Can you work these out from the model? Positions are in its coordinate system, mm. A direction names the side the tool comes from. Give positions to 0.01 mm unless a question says otherwise; leave off trailing zeros. Order: outer loops, then holes, each group sorted by start corner. A loop starts at its lowest first (then second) coordinate and runs counter-clockwise, first axis right, second up. Notation, with made-up numbers: M 30.5,69.5 L 72.5,69.5 A17 ccw 72.5,90.5 Z; hole C 48,0 d10. An arc over 180 degrees is marked long. Answer as a JSON object with one key per item and string values.
```python
from build123d import *

# Parameters (mm, degrees)
BOSS_EXTRUDE1_DEPTH               = 12.7
F_1_8_0_125_DIAMETER_HOLE1_D      = 3.175
FILLET1_R                         = 12.7
F_1_4_20_TAPPED_HOLE2_D           = 5.1054
F_1_4_20_TAPPED_HOLE2_DEPTH       = 15.875
F_1_4_20_TAPPED_HOLE2_CSINK_D     = 7.62
F_1_4_20_TAPPED_HOLE2_CSINK_ANGLE = 90
F_1_4_20_TAPPED_HOLE2_TIP         = 1.533816902
SKETCH10_W                        = 88.9
SKETCH10_H                        = 7.9375
CUT_EXTRUDE1_DEPTH                = 140.844243714


with BuildPart() as part:
    # Sketch2 → Boss-Extrude1 (new, symmetric)
    with BuildSketch(Plane.XY):
        Polygon((0, 0), (0, 95.25), (101.6, 95.25), (53.975, 47.625), (101.6, 0), align=None)
    extrude(amount=BOSS_EXTRUDE1_DEPTH, both=True)

    # 1/8 (0.125) Diameter Hole1 (through all)
    with Locations(Plane.XY.offset(12.7)):
        with Locations((53.975, 47.625)):
            Hole(F_1_8_0_125_DIAMETER_HOLE1_D / 2)

    # Fillet1
    fillet1_edges = [part.edges().sort_by_distance(p)[0] for p in [
        (0, 95.25, 0),
    ]]
    fillet(fillet1_edges, radius=FILLET1_R)

    # Sketch5 → 1/4-20 Tapped Hole1 (revolve, cut)
    with BuildSketch(Plane(origin=(6.35, 25.4, 12.7), x_dir=(0, -1, 0), z_dir=(1, 0, 0))):
        Polygon((0, 0), (0, 25.4), (3.81, 25.4), (2.5527, 24.1427), (2.5527, 1.2573), (3.81, 0), align=None)
    revolve(axis=Axis((6.35, 25.4, 19.05), (0, 0, -1)), mode=Mode.SUBTRACT)

    # 1/4-20 Tapped Hole2
    with Locations(Plane.ZY):
        with Locations((0, 41.275), (0, 9.525)):
            CounterSinkHole(F_1_4_20_TAPPED_HOLE2_D / 2, F_1_4_20_TAPPED_HOLE2_CSINK_D / 2, depth=F_1_4_20_TAPPED_HOLE2_DEPTH, counter_sink_angle=F_1_4_20_TAPPED_HOLE2_CSINK_ANGLE)
            with Locations((0, 0, -(F_1_4_20_TAPPED_HOLE2_DEPTH + F_1_4_20_TAPPED_HOLE2_TIP / 2))):  # 118° drill point
                Cone(0, F_1_4_20_TAPPED_HOLE2_D / 2, F_1_4_20_TAPPED_HOLE2_TIP, mode=Mode.SUBTRACT)

    # Sketch10 → Cut-Extrude1 (cut, through all)
    with BuildSketch(Plane(origin=(0, 95.25, 0), x_dir=(1, 0, 0), z_dir=(0, 1, 0))):
        with Locations((57.15, 8.73125)):
            Rectangle(SKETCH10_W, SKETCH10_H)
        with Locations((57.15, -8.73125)):
            Rectangle(SKETCH10_W, SKETCH10_H)
    extrude(amount=-CUT_EXTRUDE1_DEPTH, mode=Mode.SUBTRACT)


solid = part.part
```
1) I need wall thicknesses on L1, parallel to Y at x = 11.25, z = 0; L2, parallel to Y at x = 5.5, z = 0; L3, parallel to X at y = 25.5, z = -7. Which ranges of each line are inside material? Lowest first, please.
Results found:
{"L1": "y = 0 to 6.97, 12.08 to 38.72, 43.83 to 95.17", "L2": "y = 0 to 6.97, 12.08 to 22.99, 27.81 to 38.72, 43.83 to 93.01", "L3": "x = 0 to 3.8, 8.9 to 12.7"}
2) I want a section at D-D on y = 70. Write out the boundary of the cut face in (x, z).
Results found:
{"outline": "M 0,-12.7 L 12.7,-12.7 L 12.7,-4.76 L 76.35,-4.76 L 76.35,4.76 L 12.7,4.76 L 12.7,12.7 L 0,12.7 Z"}
3) I want a section at C-C on x = 6.35. Write out the boundary of the cut face in (y, z) (3 decimals), and give its area (3 significant figures).
Results found:
{"outline": "M 0,-12.7 L 21.59,-12.7 L 22.847,-11.443 L 22.847,11.443 L 21.59,12.7 L 0,12.7 Z; M 27.953,-11.443 L 29.21,-12.7 L 93.549,-12.7 L 93.549,12.7 L 29.21,12.7 L 27.953,11.443 Z; hole C 9.525,0 d5.105; hole C 41.275,0 d5.105", "area": "2,200 mm²"}
4) For faces 1 (the face through (8.668, 7.033, 0.553)), 2 (the face through (12.7, 48, 9)), 3 (the face through (78, 23.6, 0.1)), which set-ups out of +Z, -Z, +X, -X, +Y, -Y let a thin tool reach every point of the face, with its end or its side?
Results found:
{"face 1": "-X", "face 2": "+Z, +X, +Y, -Y", "face 3": "+Z, -Z, +X"}
5) I want a section at A-A on y = 25.4. Write out the boundary of the cut face in (x, z), and give its area (3 significant figures).
Results found:
{"outline": "M 0,-12.7 L 2.54,-12.7 L 3.8,-11.44 L 3.8,11.44 L 2.54,12.7 L 0,12.7 Z; M 8.9,-11.44 L 10.16,-12.7 L 12.7,-12.7 L 12.7,-4.76 L 76.2,-4.76 L 76.2,4.76 L 12.7,4.76 L 12.7,12.7 L 10.16,12.7 L 8.9,11.44 Z", "area": "795 mm²"}
6) Thinking about a two-plate mould opening in Z: for faces 4 (the face through (47, 48, -4.762)), 5 (the face through (47, 48, 4.762)), 6 (the face through (8.668, 43.806, 0.332)), 7 (the face through (78.67, 72.32, 0.07)), which applies, pulls with the +Z half, pulls with the -Z half, needs draft (parallel to the pull), parting line crosses it, or undercut?
Results found:
{"face 4": "pulls with the -Z half", "face 5": "pulls with the +Z half", "face 6": "undercut", "face 7": "needs draft"}
7) I want a section at B-B on x = 81. Write out the boundary of the cut face in (y, z), and give its area (3 significant figures).
Results found:
{"outline": "M 0,-4.76 L 20.6,-4.76 L 20.6,4.76 L 0,4.76 Z; M 74.65,-4.76 L 95.25,-4.76 L 95.25,4.76 L 74.65,4.76 Z", "area": "392 mm²"}
8) I'm going to push flat-ended pins straight in: pin 1 Ø6.5 at (y, z) = (41.275, 0) entering from +X (3 decimals); pin 2 Ø3 at (y, z) = (9.525, 0) entering from -X; pin 3 Ø2 at (x, y) = (91, 13.5) entering from -Z; pin 4 Ø8.5 at (y, z) = (61, -7) entering from +X. Where does each tip first touch, or does it pass through?
Results found:
{"pin 1": "stops at x = 63.575", "pin 2": "stops at x = 16.51", "pin 3": "passes through", "pin 4": "stops at x = 70.96"}
